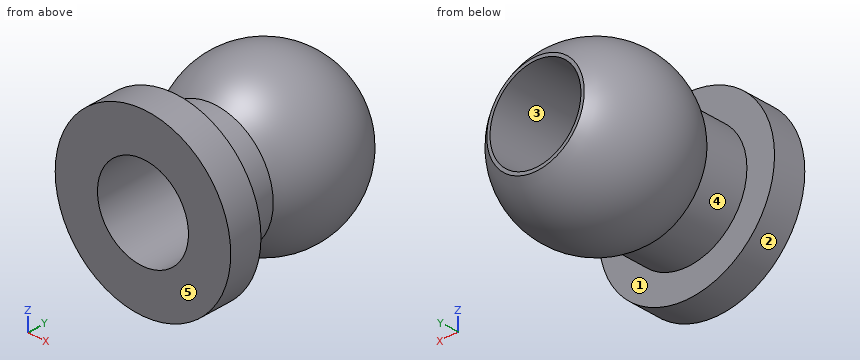
from build123d import *


with BuildPart() as part:
    # Esquisse1 → Révolution1 (revolve)
    with BuildSketch(Plane.XY, mode=Mode.PRIVATE) as r_volution1_sk:
        with BuildLine():
            Line((1.5, 2), (1.4, 2))
            Line((1.4, 2), (1.4, -4))
            Line((1.4, -4), (2.7, -4))
            Line((2.7, -4), (2.7, -3))
            Line((2.7, -3), (1.85, -3))
            Line((1.85, -3), (1.85, -1.681517172))
            ThreePointArc((1.85, -1.681517172), (2.488778249, 0.236606906), (1.5, 2))
        make_face()
    revolve(r_volution1_sk.sketch.rotate(Axis((0, 2, 0), (0, -1, 0)), 180), axis=Axis((0, 2, 0), (0, -1, 0)))


solid = part.part
Verification items for the finished model (mm, model axes). Face numbers are marked on the shaded views. A direction names the side the tool comes from. Coordinates: 2 decimals unless noted, no trailing zeros. Order: outer loops, then holes, each group sorted by start corner. A loop starts at its lowest first (then second) coordinate and runs counter-clockwise, first axis right, second up.
1. Sectioned sample at A-A, the plane x = 0. Record the cut outline in (y, z).
Results found:
outline: (-4, -2.7) - (-3, -2.7) - (-3, -1.85) - (-1.68, -1.85) arc R2.5 ccw to (2, -1.5) - (2, -1.4) - (-4, -1.4) - close; (-4, 1.4) - (2, 1.4) - (2, 1.5) arc R2.5 ccw to (-1.68, 1.85) - (-3, 1.85) - (-3, 2.7) - (-4, 2.7) - close
2. Sectioned sample at B-B, the plane z = 0. Record the cut outline in (x, y).
Results found:
outline: (-2.7, -4) - (-1.4, -4) - (-1.4, 2) - (-1.5, 2) arc R2.5 ccw to (-1.85, -1.68) - (-1.85, -3) - (-2.7, -3) - close; (1.4, -4) - (2.7, -4) - (2.7, -3) - (1.85, -3) - (1.85, -1.68) arc R2.5 ccw to (1.5, 2) - (1.4, 2) - close
3. Sectioned sample at D-D, the plane y = -3.2. Record the cut outline in (x, z), and give its area (3 significant figures).
Results found:
outline: circle Ø5.4 at (0, 0); hole circle Ø2.8 at (0, 0)
area: 16.7 mm2
4. Release check for a two-part mould opening along X. For the marked faces 1, 2 and 3 record: +X half, -X half, draft (parallel to the pull), parting line (faces both ways), or undercut.
Results found:
face 1: draft
face 2: parting line
face 3: undercut
5. Go/stop test with flat-tipped pins: pin 1 Ø2 at (y, z) = (-1, 1) entering from -X; pin 2 Ø3 at (x, z) = (0, 0) entering from -Y; pin 3 Ø2 at (y, z) = (-1, 1) entering from +X; pin 4 Ø1.7 at (x, z) = (0, 0) entering from +Y. Record where each tip stops, or that it passes through.
Results found:
pin 1: stops at x = -2.47
pin 2: stops at y = -4
pin 3: stops at x = 2.47
pin 4: passes through
6. Scan lines: line 1 (Z direction, x = 1.25, y = 1.55); line 2 (Z direction, x = 0, y = -0.5); line 3 (Y direction, x = 0.65, z = -1.8). Record each from-to range of solid material in increasing order.
Results found:
line 1: z = -1.51 to -0.63, 0.63 to 1.51
line 2: z = -2.45 to -1.4, 1.4 to 2.45
line 3: y = -4 to -3, -1.61 to 1.61
7. Set-up check for the marked faces 4 and 5: record each of +Z, -Z, +X, -X, +Y, -Y from which the full face is reachable in a straight line by a thin tool's end or side.
Results found:
face 4: none
face 5: +Z, -Z, +X, -X, -Y
8. Sectioned sample at C-C, the plane y = -2.1. Record the cut outline in (x, z).
Results found:
outline: circle Ø3.7 at (0, 0); hole circle Ø2.8 at (0, 0)
